Part model, mm, in its own coordinate system. A direction names the side the tool comes from. Round coordinates to 2 decimals unless told otherwise and drop trailing zeros. Write each loop counter-clockwise with the first axis right and the second up, starting at its lowest first coordinate (ties: lowest second). Pieces come first, ordered by that corner, then holes. Notation, with made-up numbers: M 28.5,58 L 65.5,58 A19 ccw 65.5,71 Z; hole C -34.75,-5 d1. An arc over 180 degrees is marked long. Answer as a JSON object with one key per item and string values. Group by question number.
1. Two-plate mould, pull along Z, no slides. Class faces 1 (the face through (6.26, 67.86, -33.27)), 2 (the face through (6.261, -24.59, -71.675)), 3 (the face through (12.7, -19, 1)): +Z half, -Z half, draft (parallel to the pull), parting line (faces both ways), or undercut.
2. Drop flat-ended pins along their axis: pin 1 (1.4 mm diameter, centred on x = 4, y = 7, fed in from -Z); pin 2 (2 mm diameter, centred on x = 8.5, y = -24, fed in from +Z); pin 3 (0.5 mm diameter, centred on x = 4, y = 7, fed in from +Z). Give the stop position or say it passes through.
3. Band-saw the part on B-B, the plane y = -44. Write the cut outline in (x, z).
4. Band-saw the part on A-A, the plane y = 0. Write the cut outline in (x, z), plus the area to 3 significant figures.
5. Drill centre lines: line 1 (Z direction, x = 6, y = 0); line 2 (Z direction, x = 2.75, y = 74.5); line 3 (Y direction, x = 3, z = 0). Where is each one in solid material? Low to high. Write a range as from..to.
6. Which spindle directions (+Z, -Z, +X, -X, +Y, -Y) get a long thin tool onto all of the face, cutting with end or side? Do faces 4 (the face through (6.26, -34.09, 59.14)), 5 (the face through (6.261, -75.401, -5.117)), 6 (the face through (6.439, -81.847, -10.75)), 7 (the face through (6.44, 81.84, -10.8)), 8 (the face through (6.261, 71.675, -24.59)). Say none if no direction does.
from build123d import *

# Parameters (mm, degrees)
BASPROSKE_W     = 12.7
BASPROSKE_H     = 82.55
TOOTHCUT_DEPTH  = 118.432086757
TEETHCUTS_COUNT = 24
TEETHCUTS_ANGLE = 345
BORSKE_R        = 6.35
BORE_DEPTH      = 50.8000508
KEYSKE_W        = 3.175
KEYSKE_H        = 7.874
KEYWAY_DEPTH    = 50.8000508


with BuildPart() as part:
    # BasProSke → Base-Revolve (revolve)
    with BuildSketch(Plane(origin=(0, 0, 0), x_dir=(1, 0, 0), z_dir=(0, 1, 0)), mode=Mode.PRIVATE) as base_revolve_sk:
        with Locations((6.35, 41.275)):
            Rectangle(BASPROSKE_W, BASPROSKE_H)
    revolve(base_revolve_sk.sketch.rotate(Axis((-10, 0, 0), (1, 0, 0)), 180), axis=Axis((-10, 0, 0), (1, 0, 0)))

    # TooCutSke → ToothCut (cut, through all)
    with BuildSketch(Plane(origin=(0, 0, 0), x_dir=(0, 0, -1), z_dir=(1, 0, 0))):
        with BuildLine():
            ThreePointArc((3.050766134, 68.193022716), (0, 68.26123), (-3.050766134, 68.193022716))
            ThreePointArc((-3.050766134, 68.193022716), (-5.164725154, 75.513208068), (-9.02816666, 82.080380676))
            ThreePointArc((-9.02816666, 82.080380676), (0, 82.5754), (9.02816666, 82.080380676))
            ThreePointArc((9.02816666, 82.080380676), (5.164725154, 75.513208068), (3.050766134, 68.193022716))
        make_face()
    toothcut = extrude(amount=TOOTHCUT_DEPTH, mode=Mode.SUBTRACT)

    # TeethCuts: ToothCut ×24 about axis
    teethcuts_axis = Axis((-10, 0, 0), (1, 0, 0))
    for i in range(1, TEETHCUTS_COUNT):
        add(toothcut.rotate(teethcuts_axis, i * TEETHCUTS_ANGLE / (TEETHCUTS_COUNT - 1)), mode=Mode.SUBTRACT)

    # BorSke → Bore (cut, symmetric)
    with BuildSketch(Plane(origin=(0, 0, 0), x_dir=(0, 0, -1), z_dir=(1, 0, 0))):
        with Locations(Location((0, 0, 0), (0, 0, 180))):
            Circle(BORSKE_R)
    extrude(amount=BORE_DEPTH, both=True, mode=Mode.SUBTRACT)

    # KeySke → Keyway (cut, symmetric)
    with BuildSketch(Plane(origin=(0, 0, 0), x_dir=(0, 0, -1), z_dir=(1, 0, 0))):
        with Locations((0, 3.937)):
            Rectangle(KEYSKE_W, KEYSKE_H)
    extrude(amount=KEYWAY_DEPTH, both=True, mode=Mode.SUBTRACT)


solid = part.part
Worked answers:
{
 "1": {"face 1": "undercut", "face 2": "-Z half", "face 3": "draft"},
 "2": {"pin 1": "stops at z = -80.22", "pin 2": "stops at z = 72.18", "pin 3": "stops at z = 79.51"},
 "3": {"outline": "M 0,-64.04 L 12.7,-64.04 L 12.7,64.04 L 0,64.04 Z"},
 "4": {"outline": "M 0,-68.26 L 12.7,-68.26 L 12.7,-6.35 L 0,-6.35 Z; M 0,6.35 L 12.7,6.35 L 12.7,68.26 L 0,68.26 Z", "area": "1,570 mm^2"},
 "5": {"line 1": "z = -68.26..-6.35, 6.35..68.26", "line 2": "z = -33.35..-27.14, -14.52..-4.75, 4.75..14.52, 27.14..33.35", "line 3": "y = -68.26..-6.35, 7.87..68.26"},
 "6": {"face 4": "+X, -X", "face 5": "+X, -X, -Y", "face 6": "-Z, +X, -X, -Y", "face 7": "-Z, +X, -X, +Y", "face 8": "+X, -X, +Y"}
}
